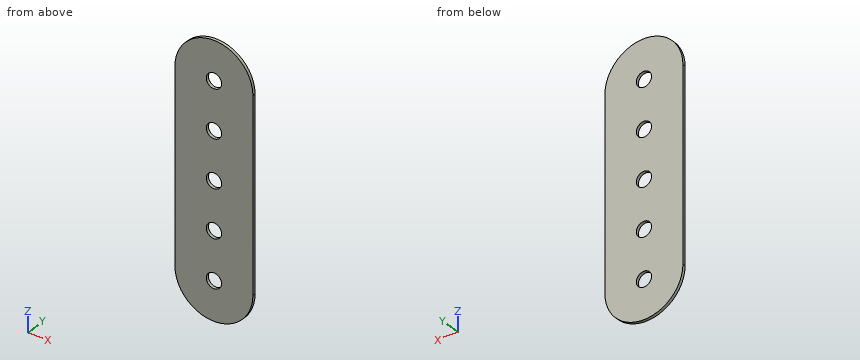
```python
from build123d import *

# Parameters (mm, degrees)
F0_R     = 2.54
F1_DEPTH = 1


with BuildPart() as f1:
    # F0 (on Front) → F1 (new body)
    with BuildSketch(Plane.XZ):
        with BuildLine():
            ThreePointArc((13, 48), (0, 35), (-13, 48))
            Line((-13, 48), (-13, -16))
            ThreePointArc((-13, -16), (0, -3), (13, -16))
            Line((13, -16), (13, 48))
        make_face()
        Circle(F0_R, mode=Mode.SUBTRACT)
        with Locations((0, 16)):
            Circle(F0_R, mode=Mode.SUBTRACT)
        with Locations((0, 32)):
            Circle(F0_R, mode=Mode.SUBTRACT)
        with BuildLine():
            ThreePointArc((13, 48), (0, 61), (-13, 48))
            ThreePointArc((-13, 48), (0, 35), (13, 48))
        make_face()
        with Locations((0, 48)):
            Circle(F0_R, mode=Mode.SUBTRACT)
        with BuildLine():
            ThreePointArc((13, -16), (0, -3), (-13, -16))
            ThreePointArc((-13, -16), (0, -29), (13, -16))
        make_face()
        with Locations((0, -16)):
            Circle(F0_R, mode=Mode.SUBTRACT)
    extrude(amount=F1_DEPTH)


solid = f1.part
```
For this review, take the finished solid that the model builds, in its own axes (mm). Round coordinates to 2 decimals unless told otherwise and drop trailing zeros. Loops run counter-clockwise (first coordinate to the right, second up) from the corner with the lowest first, then second, coordinate; pieces in that order, holes last.
(1) Wall thickness on line 1 along Z through (x, y) = (0, -0.4); line 2 along Z through (x, y) = (1, -0.6); line 3 along X through (y, z) = (-0.95, 31): over which ranges is each line inside the solid? List them lowest first.
Returned:
line 1: z = -29 to -18.54, -13.46 to -2.54, 2.54 to 13.46, 18.54 to 29.46, 34.54 to 45.46, 50.54 to 61
line 2: z = -28.96 to -18.33, -13.67 to -2.33, 2.33 to 13.67, 18.33 to 29.67, 34.33 to 45.67, 50.33 to 60.96
line 3: x = -13 to -2.33, 2.33 to 13
(2) We need section A-A (x = 0). Give the boundary of the cut face in (y, z).
Returned:
outline: (-1, -29) - (0, -29) - (0, -18.54) - (-1, -18.54) - close; (-1, -13.46) - (0, -13.46) - (0, -2.54) - (-1, -2.54) - close; (-1, 2.54) - (0, 2.54) - (0, 13.46) - (-1, 13.46) - close; (-1, 18.54) - (0, 18.54) - (0, 29.46) - (-1, 29.46) - close; (-1, 34.54) - (0, 34.54) - (0, 45.46) - (-1, 45.46) - close; (-1, 50.54) - (0, 50.54) - (0, 61) - (-1, 61) - close
(3) We need section D-D (z = -21). Give the boundary of the cut face in (x, y).
Returned:
outline: (-12, -1) - (12, -1) - (12, 0) - (-12, 0) - close
(4) We need section C-C (y = -0.65). Give the boundary of the cut face in (x, z), plus the area to 3 significant figures.
Returned:
outline: (-13, -16) arc R13 ccw to (13, -16) - (13, 48) arc R13 ccw to (-13, 48) - close; hole circle Ø5.08 at (0, -16); hole circle Ø5.08 at (0, 0); hole circle Ø5.08 at (0, 16); hole circle Ø5.08 at (0, 32); hole circle Ø5.08 at (0, 48)
area: 2,090 mm2
(5) We need section B-B (z = 32). Give the boundary of the cut face in (x, y).
Returned:
outline: (-13, -1) - (-2.54, -1) - (-2.54, 0) - (-13, 0) - close; (2.54, -1) - (13, -1) - (13, 0) - (2.54, 0) - close
(6) Clearance check with a flat-ended pin moving along its axis: P1, Ø3, axis at x = 5.5, z = 38.5, coming from the +Y side. State where the tip first meets the part, or that it passes through.
Returned:
P1: stops at y = 0
